```python
from build123d import *

# Parameters (mm, degrees)
SKETCH1_W           = 76.2
SKETCH1_H           = 19.05
BOSS_EXTRUDE1_DEPTH = 2.54
SKETCH2_W           = 60.96
SKETCH2_H           = 6.35
CUT_EXTRUDE1_DEPTH  = 2.54
FILLET1_R           = 3.175
FILLET2_R           = 1.778


with BuildPart() as part:
    # Sketch1 → Boss-Extrude1 (new body)
    with BuildSketch(Plane.XY):
        with Locations((38.1, 9.525)):
            Rectangle(SKETCH1_W, SKETCH1_H)
    extrude(amount=BOSS_EXTRUDE1_DEPTH)

    # Sketch2 → Cut-Extrude1 (cut)
    with BuildSketch(Plane.XY.offset(2.54)):
        with Locations((38.1, 9.525)):
            Rectangle(SKETCH2_W, SKETCH2_H)
    extrude(amount=-CUT_EXTRUDE1_DEPTH, mode=Mode.SUBTRACT)

    # Fillet1
    fillet1_edges = [part.edges().sort_by_distance(p)[0] for p in [
        (68.58, 6.35, 1.27),
        (7.62, 12.7, 1.27),
        (7.62, 6.35, 1.27),
        (68.58, 12.7, 1.27),
    ]]
    fillet(fillet1_edges, radius=FILLET1_R - 0.0001)  # a hair under: the kernel refuses the full size

    # Fillet2
    fillet2_edges = [part.edges().sort_by_distance(p)[0] for p in [
        (0, 19.05, 1.27),
        (76.2, 19.05, 1.27),
        (76.2, 0, 1.27),
        (0, 0, 1.27),
    ]]
    fillet(fillet2_edges, radius=FILLET2_R)


solid = part.part
```
For this review, take the finished solid that the model builds, in its own axes (mm). A direction names the side the tool comes from. Give positions to 0.01 mm unless a question says otherwise; leave off trailing zeros. Order: outer loops, then holes, each group sorted by start corner. A loop starts at its lowest first (then second) coordinate and runs counter-clockwise, first axis right, second up.
1) Take a section at A-A (x = 63.5). Give the boundary of the cut face in (y, z), then the cut area to 3 significant figures.
2) Insertion check: pin 1 (10 mm diameter, centred on x = 12.5, y = 11, fed in from -Z). The pin has a flat end and moves straight along its axis. Give the tip position at first contact, or say it passes through.
3) Take a section at C-C (y = 8). Give the boundary of the cut face in (x, z), then the cut area to 3 significant figures.
4) Wall thickness on line 1 (Y direction, x = 19.5, z = 1.15); line 2 (X direction, y = 9.75, z = 0.7); line 3 (X direction, y = 8, z = 1.95): over which ranges is each line inside the solid? List them lowest first.
5) For faces 1 (the face through (8.57, 11.79, 1.25)), 2 (the face through (38, 14, 2.54)), list the 3-axis set-ups (+Z, -Z, +X, -X, +Y, -Y) from which the entire face can be reached by the end or side of a thin tool; tool diameter is ignored.
Derived:
1. outline: (0, 0) - (6.35, 0) - (6.35, 2.54) - (0, 2.54) - close; (12.7, 0) - (19.05, 0) - (19.05, 2.54) - (12.7, 2.54) - close
1. area: 32.3 mm2
2. pin 1: stops at z = 0
3. outline: (0, 0) - (8.01, 0) - (8.01, 2.54) - (0, 2.54) - close; (68.19, 0) - (76.2, 0) - (76.2, 2.54) - (68.19, 2.54) - close
3. area: 40.7 mm2
4. line 1: y = 0 to 6.35, 12.7 to 19.05
4. line 2: x = 0 to 7.63, 68.57 to 76.2
4. line 3: x = 0 to 8.01, 68.19 to 76.2
5. face 1: +Z, -Z
5. face 2: +Z, +X, -X, +Y, -Y
